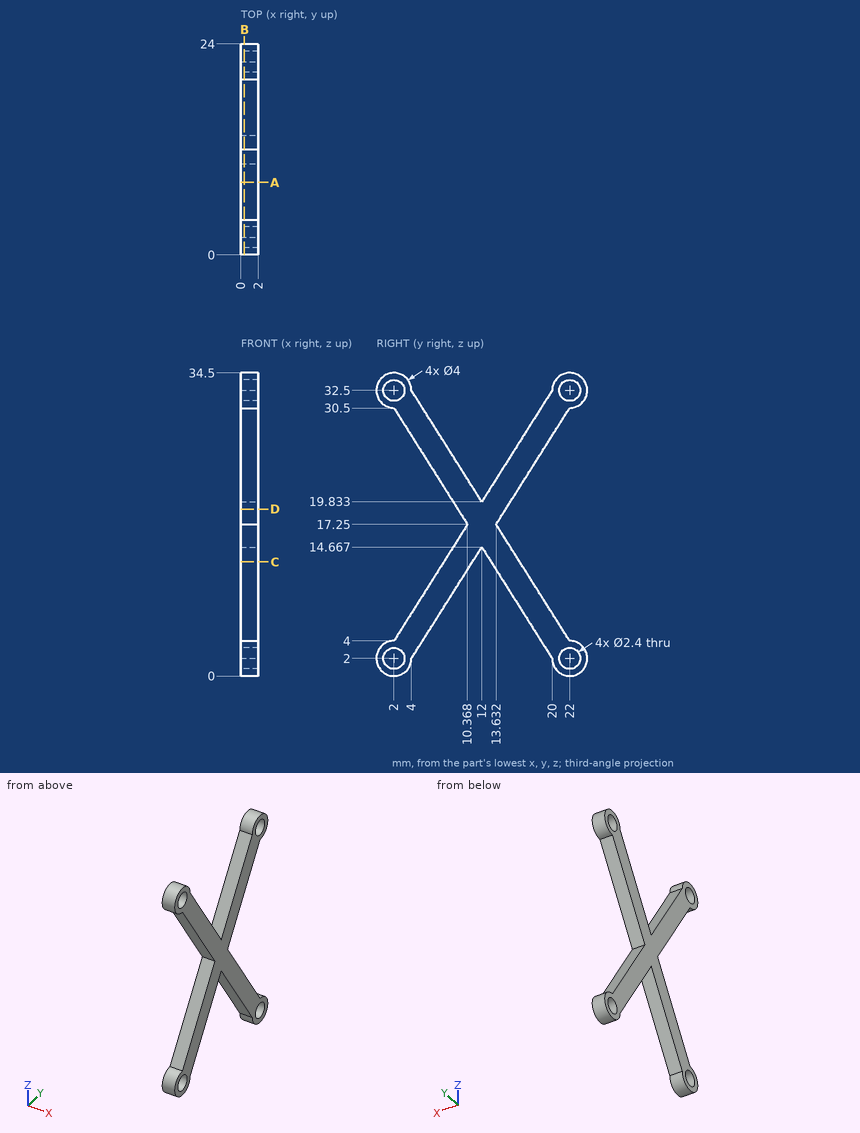
Geometry: see drawing. Coordinates: mm, zero at the bounding-box minimum. Round coordinates to 2 decimals unless told otherwise and drop trailing zeros. Order: outer loops, then holes, each group sorted by start corner. A loop starts at its lowest first (then second) coordinate and runs counter-clockwise, first axis right, second up. Notation, with made-up numbers: (28, 7) -> (74, 7) arc R17 ccw to (74, 16) -> close; hole circle Ø10 at (76, 80.25). An arc over 180 degrees is marked (long way). Use CSV: the item, a comma, the result in double quotes.
(1) Section D-D on z = 19. Return the cut outline in (x, y).
Report:
outline,"(0, 9.26) -> (2, 9.26) -> (2, 14.74) -> (0, 14.74) -> close"
(2) Section A-A on y = 8.25. Return the cut outline in (x, z) (1 decimal).
Report:
outline,"(0, 8.7) -> (2, 8.7) -> (2, 13.9) -> (0, 13.9) -> close; (0, 20.6) -> (2, 20.6) -> (2, 25.8) -> (0, 25.8) -> close"
(3) Section C-C on z = 13. Return the cut outline in (x, y) (1 decimal).
Report:
outline,"(0, 7.7) -> (2, 7.7) -> (2, 10.9) -> (0, 10.9) -> close; (0, 13.1) -> (2, 13.1) -> (2, 16.3) -> (0, 16.3) -> close"
(4) First-contact query: pin 1 Ø6 at (y, z) = (5.5, 20) entering from -X. Flat tip, straight axial feed; report the tip coordinate or a pass-through.
Report:
pin 1,"x = 0"
(5) Ray query, L1, parallel to Y at x = 1.6, z = 32.5; L2, parallel to Y at x = 0.95, z = 27.5 (1 decimal); L3, parallel to Y at x = 0.6, z = 28. Return the intervals inside material, ascending.
Report:
L1,"0 to 0.8, 3.2 to 4, 20 to 20.8, 23.2 to 24"
L2,"3.9 to 7.2, 16.8 to 20.1"
L3,"3.58 to 6.84, 17.16 to 20.42"
(6) Section B-B on x = 0.4. Return the cut outline in (y, z).
Report:
outline,"(2, 4) arc R2 ccw (long way) to (4, 2) -> (12, 14.67) -> (20, 2) arc R2 ccw (long way) to (22, 4) -> (13.63, 17.25) -> (22, 30.5) arc R2 ccw (long way) to (20, 32.5) -> (12, 19.83) -> (4, 32.5) arc R2 ccw (long way) to (2, 30.5) -> (10.37, 17.25) -> close; hole circle Ø2.4 at (2, 2); hole circle Ø2.4 at (2, 32.5); hole circle Ø2.4 at (22, 2); hole circle Ø2.4 at (22, 32.5)"
